from build123d import *

# Parameters (mm, degrees)
SKETCH1_W                                           = 23
SKETCH1_H                                           = 10
HOLE1_D                                             = 40
HOLE1_DEPTH                                         = 5.8
SKETCH4_W                                           = 12.5
SKETCH4_H                                           = 5.8
F_4_CLEARANCE_HOLE1_D                               = 3.3
F_4_CLEARANCE_HOLE1_DEPTH                           = 10
CBORE_FOR_12_BINDING_HEAD_MACHINE_SCREW_D           = 6.045
CBORE_FOR_12_BINDING_HEAD_MACHINE_SCREW_DEPTH       = 10
CBORE_FOR_12_BINDING_HEAD_MACHINE_SCREW_CBORE_D     = 11.2
CBORE_FOR_12_BINDING_HEAD_MACHINE_SCREW_CBORE_DEPTH = 6.5
FILLET1_R                                           = 5


with BuildPart() as part:
    # Sketch1 → Revolve1 (revolve)
    with BuildSketch(Plane.XZ):
        with Locations((11.5, 5)):
            Rectangle(SKETCH1_W, SKETCH1_H)
    revolve(axis=Axis((0, 0, 10), (0, 0, -1)))

    # Hole1
    with Locations(Plane(origin=(0, 0, 0), x_dir=(-1, 0, 0), z_dir=(0, 0, -1))):
        with Locations((0, 0)):
            Hole(HOLE1_D / 2, depth=HOLE1_DEPTH)

    # Sketch4 → Revolve2 (revolve)
    with BuildSketch(Plane.XZ):
        with Locations((6.25, 2.9)):
            Rectangle(SKETCH4_W, SKETCH4_H)
    revolve(axis=Axis((0, 0, 5.8), (0, 0, -1)))

    # #4 Clearance Hole1
    with Locations(Plane.XY.offset(10)):
        with Locations((14.072912811, 8.125), (14.072912811, -8.125), (0, -16.25), (-14.072912811, -8.125), (-14.072912811, 8.125), (0, 16.25)):
            Hole(F_4_CLEARANCE_HOLE1_D / 2, depth=F_4_CLEARANCE_HOLE1_DEPTH)

    # CBORE for #12 Binding Head Machine Screw1
    with Locations(Plane.XY.offset(10)):
        with Locations((0, 0)):
            CounterBoreHole(CBORE_FOR_12_BINDING_HEAD_MACHINE_SCREW_D / 2, CBORE_FOR_12_BINDING_HEAD_MACHINE_SCREW_CBORE_D / 2, CBORE_FOR_12_BINDING_HEAD_MACHINE_SCREW_CBORE_DEPTH, depth=CBORE_FOR_12_BINDING_HEAD_MACHINE_SCREW_DEPTH)

    # Fillet1
    fillet1_edges = [part.edges().sort_by_distance(p)[0] for p in [
        (-23, 0, 10),
    ]]
    fillet(fillet1_edges, radius=FILLET1_R)


solid = part.part
Check sheet for the modelled part. Datum: model origin and axes. Units: mm. A direction names the side the tool comes from. Round coordinates to 2 decimals unless told otherwise and drop trailing zeros. Write each loop counter-clockwise with the first axis right and the second up, starting at its lowest first coordinate (ties: lowest second). Pieces come first, ordered by that corner, then holes. Notation, with made-up numbers: (27.5, 75) - (34.5, 75) arc R17 cw to (34.5, 80) - close; hole circle Ø10 at (34, 56.25). An arc over 180 degrees is marked (long way). Return JSON: item names as keys, results as strings.
Q1. Cross-section at A-A (y = 0). Record the boundary of the cut face in (x, z).
Returned:
{"outline": "(-23, 0) - (-20, 0) - (-20, 5.8) - (-12.5, 5.8) - (-12.5, 0) - (-3.02, 0) - (-3.02, 3.5) - (-5.6, 3.5) - (-5.6, 10) - (-18, 10) arc R5 ccw to (-23, 5) - close; (3.02, 0) - (12.5, 0) - (12.5, 5.8) - (20, 5.8) - (20, 0) - (23, 0) - (23, 5) arc R5 ccw to (18, 10) - (5.6, 10) - (5.6, 3.5) - (3.02, 3.5) - close"}
Q2. Draft check along Y on faces 4 (the flat face through (-3, 3, 0)), 5 (the cylindrical face through (-2.994, -22.804, 2.535)), 6 (the cylindrical face through (11.923, -3.755, 2.941)). Enter one of: released by +Y, released by -Y, zero draft, split by the parting line, or undercut.
Returned:
{"face 4": "zero draft", "face 5": "split by the parting line", "face 6": "undercut"}
Q3. Cross-section at D-D (z = 9). Record the boundary of the cut face in (x, y) (3 decimals), then the cut area to 3 significant figures.
Returned:
{"outline": "circle Ø42 at (0, 0); hole circle Ø3.3 at (-14.073, -8.125); hole circle Ø3.3 at (-14.073, 8.125); hole circle Ø11.2 at (0, 0); hole circle Ø3.3 at (0, -16.25); hole circle Ø3.3 at (0, 16.25); hole circle Ø3.3 at (14.073, -8.125); hole circle Ø3.3 at (14.073, 8.125)", "area": "1,240 mm²"}
Q4. Cross-section at B-B (x = 0). Give the number of separate pieces and of enclosed holes in the cut face, then the cut area to 3 significant figures.
Returned:
{"separate pieces": "4", "enclosed holes": "0", "area": "241 mm²"}
Q5. Scan lines: L1, parallel to Y at x = 0, z = 2.3; L2, parallel to X at y = -4.5, z = 4.5; L3, parallel to Y at x = -8.5, z = 4. Record each from-to range of solid material in increasing order. Write a range as from..to.
Returned:
{"L1": "y = -23..-20, -12.5..-3.02, 3.02..12.5, 20..23", "L2": "x = -22.56..-19.49, -11.66..-3.33, 3.33..11.66, 19.49..22.56", "L3": "y = -21.37..-18.1, -9.17..9.17, 18.1..21.37"}
Q6. Depth check by flat-ended pin: P1, Ø8, axis at x = 0, y = 0, coming from the +Z side; P2, Ø4, axis at y = -4, z = 7, coming from the -X side; P3, Ø4, axis at y = 1.5, z = 8, coming from the +X side. Enter the tip coordinate at first touch or a pass-through.
Returned:
{"P1": "stops at z = 3.5", "P2": "stops at x = -22.82", "P3": "stops at x = 22.86"}
Q7. Access from +Z, -Z, +X, -X, +Y, -Y to the whole of each face (thin tool, end or side, straight path). Record for faces 1 (the cylindrical face through (-0.89, 17.64, 7.87)), 2 (the flat face through (9, 9, 5.8)), 3 (the flat face through (2.4, -2.4, 3.5)).
Returned:
{"face 1": "+Z, -Z", "face 2": "-Z", "face 3": "+Z"}
Q8. Cross-section at C-C (z = 1.25). Record the boundary of the cut face in (x, y) (1 decimal), then the cut area to 3 significant figures.
Returned:
{"outline": "circle Ø46 at (0, 0); circle Ø25 at (0, 0); hole circle Ø40 at (0, 0); hole circle Ø6 at (0, 0)", "area": "867 mm²"}
